Can you work these out from the model? Positions are in its coordinate system, mm. A direction names the side the tool comes from. Give positions to 0.01 mm unless a question says otherwise; leave off trailing zeros. Write each loop counter-clockwise with the first axis right and the second up, starting at its lowest first coordinate (ties: lowest second). Pieces come first, ordered by that corner, then holes. Notation, with made-up numbers: (-38, 55) - (0, 55) arc R8 cw to (0, 64) - close; hole circle Ø8 at (63.25, 70). An arc over 180 degrees is marked (long way). Return JSON: item names as keys, results as strings. Group by question number.
Autodesk Inventor part; units mm, degrees
ref_plane "Arbeitsebene1" through (0, 0, 22.5) normal (0, 0, 1) x (1, 0, 0)
ref_plane "YZ Plane" through (0, 0, 0) normal (1, 0, 0) x (0, 1, 0)
ref_plane "XZ Plane" through (0, 0, 0) normal (0, 1, 0) x (-1, 0, 0)
sketch "Skizze1" plane through (0, 0, 0) normal (0, 0, 1) x (1, 0, 0)
  line L0 (-25, 25) -> (25, 25)
  line L1 (25, 25) -> (25, -25)
  line L2 (25, -25) -> (-25, -25)
  line L3 (-25, -25) -> (-25, 25)
  line L4 (-35, 0) -> (35, 0)
  line L5 (0, -35) -> (0, 35)
  line L6 (21, 21) -> (-21, 21)
  line L7 (-21, 21) -> (-21, -21)
  line L8 (-21, -21) -> (21, -21)
  line L9 (21, -21) -> (21, 21)
  point P0 (0, 0)
  dimension "d0" = 50
  dimension "d1" = 50
  dimension "d2" = 4
extrude "Extrusion1" add sketch "Skizze1" along normal blind 45 contours L0 L5 L6 L7 L4 L3 | L0 L1 L4 L9 L6 L5 | L4 L7 L8 L5 L2 L3 | L1 L2 L5 L8 L9 L4
sketch "Skizze2" plane through (-25, -25, 0) normal (-1, 0, 0) x (0, 0, 1)
  line L0 (0, 50) -> (45, 50)
  line L1 (0, 0) -> (45, 0)
  line L2 (22.5, 50) -> (22.5, 0)
  line L3 (0, 46) -> (45, 46)
  line L4 (0, 4) -> (45, 4)
  line L5 (0, 46) -> (5, 46)
  line L6 (10, 41) -> (10, 9)
  line L7 (5, 4) -> (0, 4)
  line L8 (0, 4) -> (0, 46)
  line L9 (45, 4) -> (40, 4)
  line L10 (35, 9) -> (35, 41)
  line L11 (40, 46) -> (45, 46)
  line L12 (45, 46) -> (45, 4)
  arc A0 (40, 46) -> (35, 41) centre (40, 41) ccw
  arc A1 (35, 9) -> (40, 4) centre (40, 9) ccw
  arc A2 (5, 4) -> (10, 9) centre (5, 9) ccw
  arc A3 (10, 41) -> (5, 46) centre (5, 41) ccw
  point P0 (0, 25)
  point P1 (10, 4)
  point P2 (35, 46)
  dimension "d5" = 25
  dimension "d6" = 5
extrude "Extrusion2" cut sketch "Skizze2" against normal up to surface (46 mm away) contours A3 L6 A2 L4 L8 L3 | L3 L12 L4 A1 L10 A0
sketch "Skizze3" plane through (-25, 25, 0) normal (0, 1, 0) x (1, 0, 0)
  line L0 (0, -45) -> (50, -45)
  line L1 (50, 0) -> (50, -45)
  line L2 (0, 0) -> (0, -45)
  line L3 (50, -22.5) -> (0, -22.5)
  line L4 (25, -45) -> (25, 0)
  circle A0 centre (25, -22.5) radius 9
  line L5 (25, -22.5) -> (17.2058, -18)
  line L6 (25, -22.5) -> (32.7942, -18)
  point P0 (25, -31.5)
  dimension "d9" = 18
  dimension "d10" = 120
  dimension "d11" = 120
hole "Bohrung1" at (0, 25, 31.5) at (-7.7942, 25, 18) at (7.7942, 25, 18) direction (0, -1, 0) diameter 3.4 end up to surface countersink diameter 6.9 countersink angle 90
sketch "Skizze4" plane through (-25, -25, 0) normal (0, -1, 0) x (1, 0, 0)
  line L0 (50, 45) -> (0, 45)
  line L1 (0, 0) -> (0, 45)
  line L2 (50, 0) -> (50, 45)
  line L3 (0, 22.5) -> (50, 22.5)
  line L4 (25, 45) -> (25, 0)
  circle A0 centre (25, 22.5) radius 2.25
  dimension "d19" = 4.5
extrude "Extrusion3" cut sketch "Skizze4" against normal up to surface (46 mm away) contours A0 L3 L4 | L4 L3 A0 | A0 L4 L3 | L4 A0 L3
sketch "Skizze5" plane through (-25, 21, 0) normal (-1, 0, 0) x (0, 0, 1)
  circle A0 centre (22.5, -30) radius 2.25
  circle A1 centre (22.5, -12) radius 2.25
  line L0 (35, -35) -> (35, -6)
  line L1 (10, -6) -> (35, -6)
  line L2 (10, -6) -> (10, -35)
  arc A2 (5, -40) -> (10, -35) centre (5, -35) ccw
  line L3 (5, -40) -> (40, -40)
  arc A3 (35, -35) -> (40, -40) centre (40, -35) ccw
  point P0 (0, -21)
hole "Bohrung2" at (-25, 9, 22.5) at (-25, -9, 22.5) direction (1, 0, 0) diameter 3.242 end up to surface
sketch "Skizze6" plane through (0, 0, 45) normal (0, 0, 1) x (1, 0, 0)
  line L0 (-25, -25) -> (-25, -21)
  line L1 (25, -25) -> (-25, -25)
  line L2 (25, 25) -> (25, -25)
  line L3 (-25, 25) -> (25, 25)
  line L4 (-25, 21) -> (-25, 25)
  line L5 (-25, 23) -> (25, 23)
  line L6 (23, 25) -> (23, -25)
  line L7 (-25, -23) -> (25, -23)
  line L8 (-23, 25) -> (-23, -25)
  point P0 (0, 0)
  point P1 (-23, 23)
  point P2 (23, 23)
  point P3 (23, -23)
  point P4 (-23, -23)
  dimension "d29" = 2
  dimension "d30" = 2
hole "Bohrung3" at (-23, 23, 45) at (23, 23, 45) at (23, -23, 45) at (-23, -23, 45) direction (0, 0, -1) diameter 1.567 depth 8 tip angle 118
ref_plane "Arbeitsebene1" through (0, 0, 22.5) normal (0, 0, 1) x (1, 0, 0)
mirror "Spiegeln1" about plane through (0, 0, 22.5) normal (0, 0, 1) of "Bohrung3"
properties part number "1_0204_001"
1) Imagine slicing it at B-B, the plane z = 4. Write out the boundary of the cut face in (x, y).
2) On a 3-axis mill with a long thin cutter (end or side, diameter ignored), from which of +Z, -Z, +X, -X, +Y, -Y can I reach the whole of each face in a straight line? I mean faces 3 (the face through (-23, 19, 9)), 4 (the face through (-0.488, -23.028, 20.304)), 5 (the face through (21, 0, 22)), 6 (the face through (-22.972, -9.487, 24.046)). Say none if no direction works.
3) I need wall thicknesses on line 1 along Y through (x, z) = (23, 4); line 2 along X through (y, z) = (-20.5, 12.5). Which ranges of each line are inside material? Lowest first, please.
4) Imagine slicing it at A-A, the plane x = -14. Write out the boundary of the cut face in (y, z).
5) We'd pull the mould along X, two halves only. Please class faces 1 (the face through (-23, -19, 36)), 2 (the face through (23.052, 22.874, 8.389)): pulls with the +X half, pulls with the -X half, needs draft (parallel to the pull), parting line crosses it, or undercut.
6) Will these pins go through, and if not, where does the flat tip stop? pin 1 Ø0.9 at (x, y) = (23, -23) entering from +Z; pin 2 Ø1.4 at (x, y) = (-23, 23) entering from -Z; pin 3 Ø1.2 at (x, y) = (-23, 0) entering from +Z.
7) Imagine slicing it at D-D, the plane z = 12. Write out the boundary of the cut face in (x, y), and give its area (3 significant figures).
8) Imagine slicing it at C-C, the plane y = 12. Write out the boundary of the cut face in (x, z).
Resolved:
{
 "1": {"outline": "(-25, -25) - (25, -25) - (25, 25) - (-25, 25) - (-25, 21) - (21, 21) - (21, -21) - (-25, -21) - close; hole circle Ø1.57 at (-23, -23); hole circle Ø1.57 at (-23, 23); hole circle Ø1.57 at (23, -23); hole circle Ø1.57 at (23, 23)"},
 "2": {"face 3": "-Z, -X", "face 4": "-Y", "face 5": "+Z, -Z", "face 6": "-X"},
 "3": {"line 1": "-25 to -23.78, -22.22 to 22.22, 23.78 to 25", "line 2": "-25 to -21, 21 to 25"},
 "4": {"outline": "(-25, 0) - (-21, 0) - (-21, 45) - (-25, 45) - close; (21, 0) - (25, 0) - (25, 45) - (21, 45) - close"},
 "5": {"face 1": "needs draft", "face 2": "undercut"},
 "6": {"pin 1": "z = 36.8", "pin 2": "z = 8.05", "pin 3": "z = 35"},
 "7": {"outline": "(-25, -25) - (25, -25) - (25, 25) - (-25, 25) - close; hole (-21, -21) - (21, -21) - (21, 21) - (-21, 21) - close", "area": "736 mm^2"},
 "8": {"outline": "(-25, 10) - (-21, 10) - (-21, 35) - (-25, 35) - close; (21, 0) - (25, 0) - (25, 45) - (21, 45) - close"}
}
